Model file for the job. Use its own axes, mm. Face numbers are marked on the shaded views. Round coordinates to 2 decimals unless told otherwise and drop trailing zeros. Order: outer loops, then holes, each group sorted by start corner. A loop starts at its lowest first (then second) coordinate and runs counter-clockwise, first axis right, second up. Notation, with made-up numbers: (75, 67) -> (94, 67) arc R14 ccw to (94, 86) -> close; hole circle Ø1 at (17, 84.5). An arc over 180 degrees is marked (long way). Answer as CSV lines item,"result".
```python
from build123d import *

# Parameters (mm, degrees)
EXTRUDE_1_DEPTH     = 10
SKETCH_3_R          = 5
EXTRUDE_2_DEPTH     = 2
CHAMFER_1_SIZE      = 2
CHAMFER_2_SIZE      = 2
SKETCH_4_R          = 2.1
SKETCH_4_R_2        = 3.1
CUT_EXTRUDE_1_DEPTH = 72.161787499
FILLET_1_R          = 1


with BuildPart() as part:
    # 草图1 → 凸台-拉伸1 (new, symmetric)
    with BuildSketch(Plane.XY):
        Polygon((0, 4), (0, 10), (70, 10), (70, 2), (30, 2), (30, 4), align=None)
    extrude(amount=EXTRUDE_1_DEPTH, both=True)

    # 草图3 → 凸台-拉伸2 (add)
    with BuildSketch(Plane.XZ.offset(-4)):
        with Locations(Location((8, 0, 0), (0, 0, 90))):
            Circle(SKETCH_3_R)
    extrude(amount=EXTRUDE_2_DEPTH)

    # 倒角1
    chamfer_1_edges = [part.edges().sort_by_distance(p)[0] for p in [
        (0, 7, -10),
        (0, 7, 10),
    ]]
    chamfer(chamfer_1_edges, length=CHAMFER_1_SIZE)

    # 倒角2
    chamfer_2_edges = [part.edges().sort_by_distance(p)[0] for p in [
        (70, 6, 10),
        (70, 6, -10),
    ]]
    chamfer(chamfer_2_edges, length=CHAMFER_2_SIZE)

    # 草图4 → 切除-拉伸1 (cut, through all)
    with BuildSketch(Plane.XZ.offset(-2)):
        with Locations((40, 0)):
            Circle(SKETCH_4_R)
        with Locations((60, 0)):
            Circle(SKETCH_4_R)
        with Locations((8, 0)):
            Circle(SKETCH_4_R_2)
    extrude(amount=-CUT_EXTRUDE_1_DEPTH, mode=Mode.SUBTRACT)

    # 圆角1
    fillet_1_edges = [part.edges().sort_by_distance(p)[0] for p in [
        (8, 4, -5),
    ]]
    fillet(fillet_1_edges, radius=FILLET_1_R)


solid = part.part
```
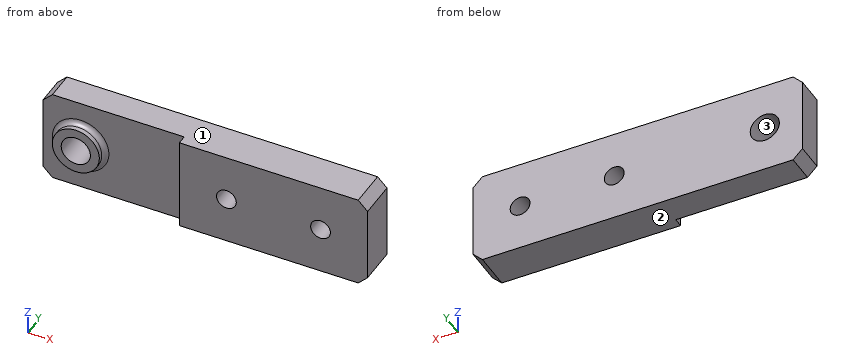
Q1. Wall check: L1, parallel to X at y = 3.25, z = -1; L2, parallel to Z at x = 60, y = 8; L3, parallel to X at y = 8.75, z = -0.75. Give the ranges that are in metal, low to high. Write a range as [from, to].
Checks:
L1,"[3.07, 5.07], [10.93, 12.93], [30, 38.15], [41.85, 58.15], [61.85, 70]"
L2,"[-10, -2.1], [2.1, 10]"
L3,"[0, 4.99], [11.01, 38.04], [41.96, 58.04], [61.96, 70]"
Q2. Saw through at D-D (x = 8). Write the cut outline in (y, z).
Checks:
outline,"(2, -5) -> (3, -5) arc R1 cw to (4, -6) -> (4, -10) -> (10, -10) -> (10, -3.1) -> (2, -3.1) -> close; (2, 3.1) -> (10, 3.1) -> (10, 10) -> (4, 10) -> (4, 6) arc R1 cw to (3, 5) -> (2, 5) -> close"
Q3. Saw through at C-C (y = 9.25). Write the cut outline in (x, z), plus the area to 3 significant figures.
Checks:
outline,"(0, -8) -> (2, -10) -> (68, -10) -> (70, -8) -> (70, 8) -> (68, 10) -> (2, 10) -> (0, 8) -> close; hole circle Ø6.2 at (8, 0); hole circle Ø4.2 at (40, 0); hole circle Ø4.2 at (60, 0)"
area,"1,330 mm²"
Q4. Mould opens along Z. For the marked faces 1, 2 and 3 say: +Z half, -Z half, draft (parallel to the pull), parting line (faces both ways), or undercut.
Checks:
face 1,"+Z half"
face 2,"-Z half"
face 3,"undercut"
Q5. Saw through at B-B (x = 60). Write the cut outline in (y, z), plus the area to 3 significant figures.
Checks:
outline,"(2, -10) -> (10, -10) -> (10, -2.1) -> (2, -2.1) -> close; (2, 2.1) -> (10, 2.1) -> (10, 10) -> (2, 10) -> close"
area,"126 mm²"
Q6. Saw through at A-A (z = 0). Write the cut outline in (x, y), plus the area to 3 significant figures.
Checks:
outline,"(0, 4) -> (2, 4) arc R1 cw to (3, 3) -> (3, 2) -> (4.9, 2) -> (4.9, 10) -> (0, 10) -> close; (11.1, 2) -> (13, 2) -> (13, 3) arc R1 cw to (14, 4) -> (30, 4) -> (30, 2) -> (37.9, 2) -> (37.9, 10) -> (11.1, 10) -> close; (42.1, 2) -> (57.9, 2) -> (57.9, 10) -> (42.1, 10) -> close; (62.1, 2) -> (70, 2) -> (70, 10) -> (62.1, 10) -> close"
area,"404 mm²"
